Here's how the part is built. I have some questions about the finished solid (model axes, mm). Round coordinates to 2 decimals unless told otherwise and drop trailing zeros. Use a Markdown table: item, result. Add a question column.
```python
from build123d import *

# Parameters (mm, degrees)
SKETCH1_R             = 4.7625
SKETCH1_R_2           = 3.175
BOSS_EXTRUDE1_DEPTH   = 6.35
BOSS_EXTRUDE1_2_DEPTH = 6.35
SKETCH2_R             = 4.7625
SKETCH2_R_2           = 3.175
REVOLVE1_ANGLE        = 180


with BuildPart() as part:
    # Sketch1 → Boss-Extrude1 (new body)
    with BuildSketch(Plane(origin=(0, 0, 0), x_dir=(0, 0, -1), z_dir=(1, 0, 0))):
        Circle(SKETCH1_R)
        Circle(SKETCH1_R_2, mode=Mode.SUBTRACT)
    extrude(amount=BOSS_EXTRUDE1_DEPTH)



with BuildPart() as body_2:
    # Sketch1 → Boss-Extrude1 2 (new body)
    with BuildSketch(Plane(origin=(0, 0, 0), x_dir=(0, 0, -1), z_dir=(1, 0, 0))):
        with Locations((30.48, 0)):
            Circle(SKETCH1_R)
        with Locations((30.48, 0)):
            Circle(SKETCH1_R_2, mode=Mode.SUBTRACT)
    extrude(amount=BOSS_EXTRUDE1_2_DEPTH)


with BuildPart() as part_1:
    add(part.part)

    add(body_2.part)  # Revolve1 merges body 2
    # Sketch2 → Revolve1 (revolve)
    with BuildSketch(Plane(origin=(6.35, 0, 0), x_dir=(0, 0, -1), z_dir=(1, 0, 0))):
        with Locations(Location((0, 0, 0), (0, 0, 180))):
            Circle(SKETCH2_R)
        with Locations(Location((0, 0, 0), (0, 0, 180))):
            Circle(SKETCH2_R_2, mode=Mode.SUBTRACT)
    revolve(axis=Axis((6.35, 0, -15.24), (0, 1, 0)), revolution_arc=REVOLVE1_ANGLE)


solid = part_1.part
```
Item 1: Imagine slicing it at B-B on x = 16.25. Count the separate pieces of the cut face and the enclosed holes in it, plus the area to 3 significant figures.
Item 2: For pin 1 Ø5 at (x, y) = (15.5, 2.5) entering from -Z; pin 2 Ø1.5 at (y, z) = (-3, -10) entering from +X; pin 3 Ø2 at (y, z) = (-3.5, -9.5) entering from -X, each with a flat end and sliding along its axis, tell me the tip position at first contact or that it passes through.
Item 3: I need wall thicknesses on probe 1 along Y at (x, z) = (4.25, 0) (1 decimal); probe 2 along Z at (x, y) = (3.75, 2.5); probe 3 along Y at (x, z) = (12.5, -4). Which ranges of each line are inside material? Lowest first, please. Write a range as from..to.
Item 4: If we mould it in two halves opening along Z, with no side actions, what happens to faces 1 (the face through (0, -1, -34)), 2 (the face through (3.13, 0.95, -33.51))? For each: +Z half, -Z half, draft (parallel to the pull), parting line (faces both ways), or undercut.
The answers:
| question | item | result |
|---|---|---|
| 1 | separate pieces | 2 |
| 1 | enclosed holes | 2 |
| 1 | area | 116 mm² |
| 2 | pin 1 | z = -33.81 |
| 2 | pin 2 | x = 25.11 |
| 2 | pin 3 | x = 15.72 |
| 3 | probe 1 | -4.8..-3.2, 3.2..4.8 |
| 3 | probe 2 | -34.53..-32.44, -28.52..-26.43, -4.05..-1.96, 1.96..4.05 |
| 3 | probe 3 | -4.1..-2.05, 2.05..4.1 |
| 4 | face 1 | draft |
| 4 | face 2 | undercut |
